from build123d import *

# Parameters (mm, degrees)
F0_R     = 73.2317789394
F1_DEPTH = 25.4
F2_DEPTH = 25.4
F4_T     = -2.54
F3_W     = 73.9012621343
F3_H     = 74.8767629266
F5_DEPTH = 51.816
F6_R     = 5.08


with BuildPart() as f1:
    # F0 (on Right) → F1 (new body)
    with BuildSketch(Plane.YZ):
        Circle(F0_R)
    extrude(amount=F1_DEPTH)

    # F2 (add): a face of the model
    f2_faces = [f1.faces().sort_by_distance(p)[0] for p in [
        (25.4, 0, 0),
    ]]
    extrude(f2_faces, amount=F2_DEPTH)

    # F4
    f4_openings = [f1.faces().sort_by_distance(p)[0] for p in [
        (50.8, 0, 0),
    ]]
    offset(amount=F4_T, openings=f4_openings)

    # F3 (on face) → F5 (join)
    with BuildSketch(Plane.YZ.offset(50.8)):
        with Locations((-3.3096689731, 2.6898309588)):
            Rectangle(F3_W, F3_H)
    extrude(amount=-F5_DEPTH)

    # F6
    f6_edges = [f1.edges().sort_by_distance(p)[0] for p in [
        (50.8, -3.309669, 40.128212),
        (50.8, -40.2603, 2.689831),
        (50.8, 33.640962, 2.689831),
        (50.8, -3.309669, -34.748551),
    ]]
    fillet(f6_edges, radius=F6_R)


solid = f1.part
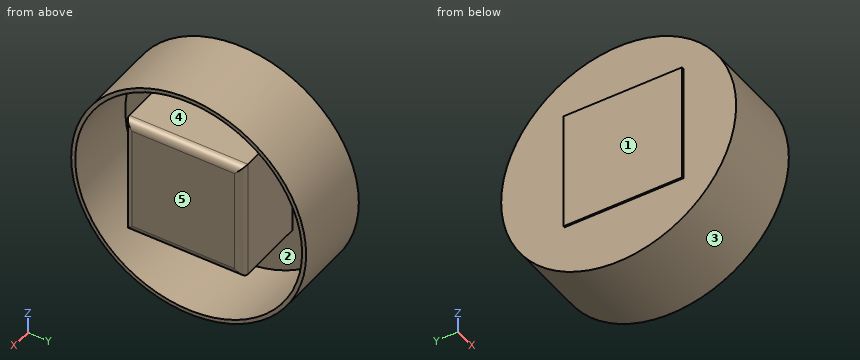
For this review, take the finished solid that the model builds, in its own axes (mm). Face numbers are marked on the shaded views. A direction names the side the tool comes from. Coordinates: 2 decimals unless noted, no trailing zeros. Order: outer loops, then holes, each group sorted by start corner. A loop starts at its lowest first (then second) coordinate and runs counter-clockwise, first axis right, second up. Notation, with made-up numbers: (13.25, 64.5) -> (47.25, 64.5) arc R23 ccw to (47.25, 98.5) -> close; hole circle Ø8 at (-35.75, -30.75). An arc over 180 degrees is marked (long way). Return JSON: item names as keys, results as strings.
1. For line 1 (Z direction, x = 21, y = 0); line 2 (Y direction, x = 13.5, z = -17); line 3 (Z direction, x = 10.5, y = -30.5), list the stretches that pass through material, from the lowest coordinate up. Write a range as from..to.
Answer block:
{"line 1": "-73.23..-70.69, -34.75..40.13, 70.69..73.23", "line 2": "-71.23..-68.62, -40.26..33.64, 68.62..71.23", "line 3": "-66.58..-63.77, -34.75..40.13, 63.77..66.58"}
2. We need section C-C on z = 0. Write out the cut boundary in (x, y), and give its area (3 significant figures).
Answer block:
{"outline": "(-1.02, -40.26) -> (0, -40.26) -> (0, -73.23) -> (50.8, -73.23) -> (50.8, -70.69) -> (2.54, -70.69) -> (2.54, -40.26) -> (45.72, -40.26) arc R5.08 ccw to (50.8, -35.18) -> (50.8, 28.56) arc R5.08 ccw to (45.72, 33.64) -> (2.54, 33.64) -> (2.54, 70.69) -> (50.8, 70.69) -> (50.8, 73.23) -> (0, 73.23) -> (0, 33.64) -> (-1.02, 33.64) -> close", "area": "4,250 mm²"}
3. We need section D-D on y = -48.5. Write out the cut boundary in (x, z).
Answer block:
{"outline": "(0, -54.87) -> (50.8, -54.87) -> (50.8, -51.43) -> (2.54, -51.43) -> (2.54, 51.43) -> (50.8, 51.43) -> (50.8, 54.87) -> (0, 54.87) -> close"}
4. Machinability: for the marked faces 4 and 5, which of the approach directions +Z, -Z, +X, -X, +Y, -Y give a long, thin tool a straight path to every point of the face, cutting with its end or side? Answer none if there is none.
Answer block:
{"face 4": "+X", "face 5": "+Z, -Z, +X, +Y, -Y"}
5. For pin 1 Ø5 at (x, y) = (7, 32) entering from -Z; pin 2 Ø1.5 at (y, z) = (-55.5, 23) entering from -X; pin 3 Ø21.5 at (x, z) = (25.5, -14) entering from -Y, all flat-tipped, find the tip position at first contact; note any pin that passes through.
Answer block:
{"pin 1": "z = -67.03", "pin 2": "x = 0", "pin 3": "y = -73.16"}
6. The part is to be moulded in two halves that separate along Y. For the marked faces 1, 2 and 3, say which applies: +Y half, -Y half, draft (parallel to the pull), parting line (faces both ways), or undercut.
Answer block:
{"face 1": "draft", "face 2": "undercut", "face 3": "parting line"}
7. We need section A-A on x = 17.5. Write out the cut boundary in (y, z).
Answer block:
{"outline": "circle Ø146.46 at (0, 0); (-40.26, -34.75) -> (33.64, -34.75) -> (33.64, 40.13) -> (-40.26, 40.13) -> close; hole circle Ø141.38 at (0, 0)"}
8. We need section B-B on y = 0. Write out the cut boundary in (x, z).
Answer block:
{"outline": "(-1.02, -34.75) -> (0, -34.75) -> (0, -73.23) -> (50.8, -73.23) -> (50.8, -70.69) -> (2.54, -70.69) -> (2.54, -34.75) -> (45.72, -34.75) arc R5.08 ccw to (50.8, -29.67) -> (50.8, 35.05) arc R5.08 ccw to (45.72, 40.13) -> (2.54, 40.13) -> (2.54, 70.69) -> (50.8, 70.69) -> (50.8, 73.23) -> (0, 73.23) -> (0, 40.13) -> (-1.02, 40.13) -> close"}
